Job drawing, mm, ordinate dimensions from the low corner. One solid piece. Coordinates: 2 decimals unless noted, no trailing zeros. Write each loop counter-clockwise with the first axis right and the second up, starting at its lowest first coordinate (ties: lowest second). Pieces come first, ordered by that corner, then holes. Notation, with made-up numbers: (37, -32) -> (92, -32) arc R25 ccw to (92, -19) -> close; hole circle Ø10 at (-24.75, 0). An arc over 180 degrees is marked (long way). One line per question, with ' | ' between items. Start each with the question number.
Item 1: Saw through at A-A (z = 4.5). List the corners of the cut face in (x, y) (3 decimals).
Item 2: Saw through at B-B (x = 373). List the corners of the cut face in (y, z).
Item 3: Probe probe 1 along X at (y, z) = (199.5, 8.5) (3 decimals); probe 2 along Y at (x, z) = (547, 6.5). List the from-to ranges inside material, lowest first. Write a range as [from, to].
Item 4: Saw through at C-C (y = 712). List the corners of the cut face in (x, z) (3 decimals).
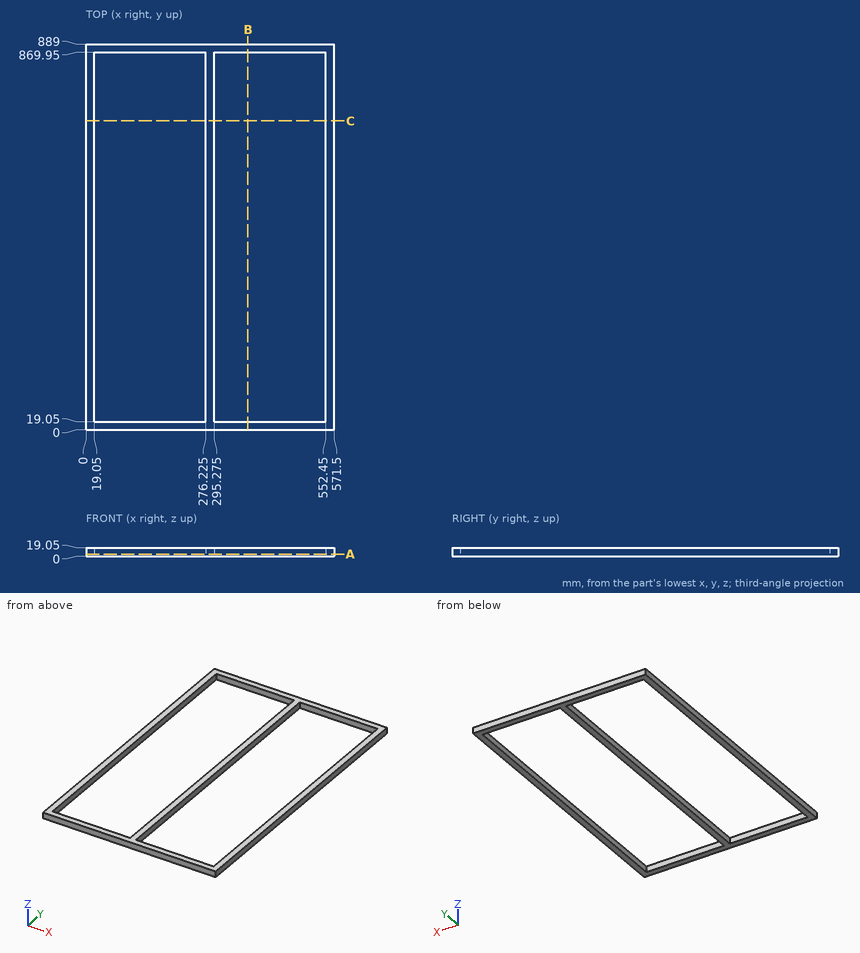
From the geometry:
1) outline: (0, 0) -> (571.5, 0) -> (571.5, 889) -> (0, 889) -> close; hole (19.05, 19.05) -> (276.225, 19.05) -> (276.225, 869.95) -> (19.05, 869.95) -> close; hole (295.275, 19.05) -> (552.45, 19.05) -> (552.45, 869.95) -> (295.275, 869.95) -> close
2) outline: (0, 0) -> (19.05, 0) -> (19.05, 19.05) -> (0, 19.05) -> close; (869.95, 0) -> (889, 0) -> (889, 19.05) -> (869.95, 19.05) -> close
3) probe 1: [0, 19.05], [276.225, 295.275], [552.45, 571.5] | probe 2: [0, 19.05], [869.95, 889]
4) outline: (0, 0) -> (19.05, 0) -> (19.05, 19.05) -> (0, 19.05) -> close; (276.225, 0) -> (295.275, 0) -> (295.275, 19.05) -> (276.225, 19.05) -> close; (552.45, 0) -> (571.5, 0) -> (571.5, 19.05) -> (552.45, 19.05) -> close
